from build123d import *

# Parameters (mm, degrees)
SALIENTE_EXTRUIR1_DEPTH    = 10
CROQUIS2_R                 = 7.5
CORTAR_EXTRUIR1_DEPTH      = 1
CORTAR_EXTRUIR1_DEPTH_BACK = 21
CROQUIS3_R                 = 7.5
CORTAR_EXTRUIR2_DEPTH      = 1
CORTAR_EXTRUIR2_DEPTH_BACK = 21


with BuildPart() as part:
    # Croquis1 → Saliente-Extruir1 (new body, symmetric)
    with BuildSketch(Plane.XY):
        Polygon((0, 11.759082218), (46.5, 11.759082218), (46.5, -8.240917782), (-46.5, -8.240917782), (-46.5, 11.759082218), align=None)
    extrude(amount=SALIENTE_EXTRUIR1_DEPTH, both=True)

    # Croquis2 → Cortar-Extruir1 (cut, two sides)
    with BuildSketch(Plane.XY.offset(10)) as cortar_extruir1_sk:
        with Locations((36.5, 1.759082218)):
            Circle(CROQUIS2_R)
    extrude(amount=CORTAR_EXTRUIR1_DEPTH, mode=Mode.SUBTRACT)
    extrude(cortar_extruir1_sk.sketch, amount=-CORTAR_EXTRUIR1_DEPTH_BACK, mode=Mode.SUBTRACT)

    # Croquis3 → Cortar-Extruir2 (cut, two sides)
    with BuildSketch(Plane(origin=(0, 11.759082218, 0), x_dir=(1, 0, 0), z_dir=(0, 1, 0))) as cortar_extruir2_sk:
        with Locations((-36.5, 0)):
            Circle(CROQUIS3_R)
    extrude(amount=CORTAR_EXTRUIR2_DEPTH, mode=Mode.SUBTRACT)
    extrude(cortar_extruir2_sk.sketch, amount=-CORTAR_EXTRUIR2_DEPTH_BACK, mode=Mode.SUBTRACT)


solid = part.part
Could you check a few things on this model? Use its own coordinates, in mm. Give positions to 0.01 mm unless a question says otherwise; leave off trailing zeros. Order: outer loops, then holes, each group sorted by start corner. A loop starts at its lowest first (then second) coordinate and runs counter-clockwise, first axis right, second up.
Item 1: I need wall thicknesses on line 1 (Y direction, x = 36.5, z = -4.5); line 2 (Z direction, x = -36.5, y = -2); line 3 (X direction, y = -6.5, z = 0.5). Which ranges of each line are inside material? Lowest first, please.
Item 2: If we mould it in two halves opening along X, with no side actions, what happens to faces 1 (the face through (1, 11.759, 0)), 2 (the face through (-44, 2, 0)), 3 (the face through (46.5, 2, 0))? For each: pulls with the +X half, pulls with the -X half, needs draft (parallel to the pull), parting line crosses it, or undercut.
Item 3: If we section it at C-C, the plane z = 0: Write out the boundary of the cut face in (x, y), plus the area to 3 significant figures.
Item 4: If we section it at A-A, the plane z = -6.5: Write out the boundary of the cut face in (x, y), plus the area to 3 significant figures.
Item 5: If we section it at B-B, the plane x = -36.5: Write out the boundary of the cut face in (y, z).
Values:
1. line 1: y = -8.24 to -5.74, 9.26 to 11.76
1. line 2: z = -10 to -7.5, 7.5 to 10
1. line 3: x = -46.5 to -43.98, -29.02 to 46.5
2. face 1: needs draft
2. face 2: undercut
2. face 3: pulls with the +X half
3. outline: (-46.5, -8.24) - (-44, -8.24) - (-44, 11.76) - (-46.5, 11.76) - close; (-29, -8.24) - (46.5, -8.24) - (46.5, 11.76) - (-29, 11.76) - close; hole circle Ø15 at (36.5, 1.76)
3. area: 1,380 mm2
4. outline: (-46.5, -8.24) - (-40.24, -8.24) - (-40.24, 11.76) - (-46.5, 11.76) - close; (-32.76, -8.24) - (46.5, -8.24) - (46.5, 11.76) - (-32.76, 11.76) - close; hole circle Ø15 at (36.5, 1.76)
4. area: 1,530 mm2
5. outline: (-8.24, -10) - (11.76, -10) - (11.76, -7.5) - (-8.24, -7.5) - close; (-8.24, 7.5) - (11.76, 7.5) - (11.76, 10) - (-8.24, 10) - close
